```python
from build123d import *

# Parameters (mm, degrees)
F0_R     = 6
F1_DEPTH = 46
F2_W     = 26.921937
F2_H     = 36
F3_DEPTH = 42.5


with BuildPart() as f1:
    # F0 (on Front) → F1 (new body)
    with BuildSketch(Plane.XZ):
        with BuildLine():
            Line((-9, 44.998586), (-15, 44.998586))
            Line((-15, 44.998586), (-15, 22.998586))
            Line((-15, 22.998586), (-5, 22.998586))
            Line((-5, 22.998586), (-5, -26.177896))
            Line((-5, -26.177896), (5, -26.177896))
            Line((5, -26.177896), (13, -26.177896))
            ThreePointArc((13, -26.177896), (24, -15.177896), (13, -4.177896))
            Line((13, -4.177896), (5, -4.177896))
            Line((5, -4.177896), (5, 22.998586))
            Line((5, 22.998586), (15, 22.998586))
            Line((15, 22.998586), (15, 44.998586))
            Line((15, 44.998586), (9, 44.998586))
            Line((9, 44.998586), (9, 28.998586))
            Line((9, 28.998586), (-9, 28.998586))
            Line((-9, 28.998586), (-9, 44.998586))
        make_face()
        with Locations((13, -15.177896)):
            Circle(F0_R, mode=Mode.SUBTRACT)
    extrude(amount=F1_DEPTH)


with BuildPart() as f3:
    # F2 (on face) → F3 (new body)
    with BuildSketch(Plane(origin=(0, 0, -26.177896), x_dir=(1, 0, 0), z_dir=(0, 0, -1))):
        with Locations((18.460968, 23)):
            Rectangle(F2_W, F2_H)
    extrude(amount=-F3_DEPTH)


with BuildPart() as f1_1:
    add(f1.part)

    # F4: cut F3
    add(f3.part, mode=Mode.SUBTRACT)


solid = f1_1.part
```
CAD build for the part. Positions are in the model's coordinates, mm. A direction names the side the tool comes from. Round coordinates to 2 decimals unless told otherwise and drop trailing zeros. Order: outer loops, then holes, each group sorted by start corner. A loop starts at its lowest first (then second) coordinate and runs counter-clockwise, first axis right, second up.
Item 1: Mould opens along Y. For faces 1 (the face through (4, -46, 2)), 2 (the face through (24, -43, -15)), 3 (the face through (19, -5, -18)) say: pulls with the +Y half, pulls with the -Y half, needs draft (parallel to the pull), parting line crosses it, or undercut.
Item 2: Tool access for faces 4 (the face through (9, -43, -4.178)), 5 (the face through (19, -41, -18)), 6 (the face through (-5, -23, -1)), 7 (the face through (0, -23, 28.999)), 8 (the face through (15, -23, 34)): list every direction of +Z, -Z, +X, -X, +Y, -Y with a clear straight run to the whole face (end or side of a thin tool).
Item 3: Probe line 1 along Z through (x, y) = (13, -2.55); line 2 along Z through (x, y) = (14.5, -2.5); line 3 along X through (y, z) = (-17.5, -9.5). List the from-to ranges inside material, lowest first.
Item 4: Saw through at B-B on x = 20. Write the cut outline in (y, z).
Item 5: Pin check, flat tips, straight feed: pin 1 (12 mm diameter, centred on x = 4, z = 31.5, fed in from +Y); pin 2 (5 mm diameter, centred on x = -8.5, y = -7, fed in from -Z); pin 3 (5 mm diameter, centred on y = -11.5, z = -2.5, fed in from +X); pin 4 (17.5 mm diameter, centred on y = -32, z = 34, fed in from +X). Stop position of each tip, or through.
Item 6: Saw through at D-D on z = 2. Write the cut outline in (x, y).
Item 7: Saw through at C-C on y = -18. Write the cut outline in (x, z), then the cut area to 3 significant figures.
Item 8: Saw through at A-A on z = 39. Write the cut outline in (x, y).
Reported:
1. face 1: pulls with the -Y half
1. face 2: needs draft
1. face 3: undercut
2. face 4: +X, +Y, -Y
2. face 5: -Z, +X
2. face 6: -Z, -X, +Y, -Y
2. face 7: +Z, +Y, -Y
2. face 8: +Z, +X, +Y, -Y
3. line 1: z = -26.18 to -21.18, -9.18 to -4.18, 23 to 45
3. line 2: z = -26.08 to -20.99, -9.37 to -4.28, 23 to 45
3. line 3: x = -5 to 5
4. outline: (-46, -23.66) - (-41, -23.66) - (-41, -6.69) - (-46, -6.69) - close; (-5, -23.66) - (0, -23.66) - (0, -6.69) - (-5, -6.69) - close
5. pin 1: stops at y = 0
5. pin 2: stops at z = 23
5. pin 3: stops at x = 5
5. pin 4: stops at x = 15
6. outline: (-5, -46) - (5, -46) - (5, 0) - (-5, 0) - close
7. outline: (-15, 23) - (-5, 23) - (-5, -26.18) - (5, -26.18) - (5, 23) - (15, 23) - (15, 45) - (9, 45) - (9, 29) - (-9, 29) - (-9, 45) - (-15, 45) - close
7. area: 864 mm2
8. outline: (-15, -46) - (-9, -46) - (-9, 0) - (-15, 0) - close; (9, -46) - (15, -46) - (15, 0) - (9, 0) - close
